Geometry check sheet. Reference: the model listing, model coordinates, mm. Face numbers are marked on the shaded views. Round coordinates to 2 decimals unless told otherwise and drop trailing zeros. Loops run counter-clockwise (first coordinate to the right, second up) from the corner with the lowest first, then second, coordinate; pieces in that order, holes last. Notation, with made-up numbers: M -40,77 L 8,77 A27 cw 8,96 Z; hole C 6.25,62 d5. An arc over 180 degrees is marked long. Write item = value, one per line.
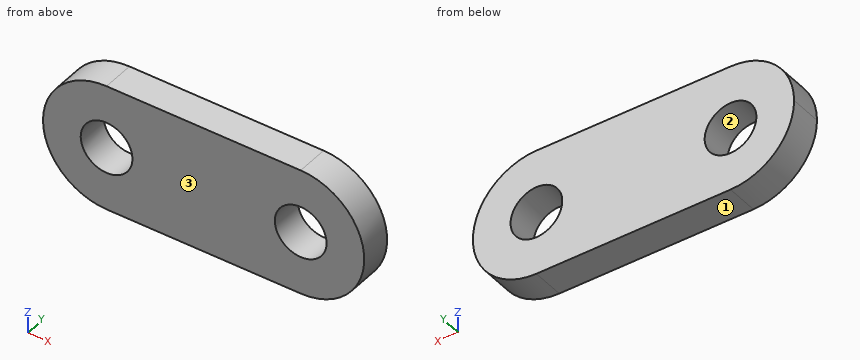
from build123d import *

# Parameters (mm, degrees)
F0_R     = 4.0005
F1_DEPTH = 2.5


with BuildPart() as f1:
    # F0 (on Front) → F1 (new body, symmetric)
    with BuildSketch(Plane.XZ):
        with BuildLine():
            Line((0, 9.8298), (0, 0))
            Line((0, 0), (-11.0109, 0))
            ThreePointArc((-11.0109, 0), (-15.0114, -4.0005), (-19.0119, 0))
            Line((-19.0119, 0), (-24.8412, 0))
            ThreePointArc((-24.8412, 0), (-21.962118, -6.950718), (-15.0114, -9.8298))
            Line((-15.0114, -9.8298), (0, -9.8298))
            Line((0, -9.8298), (15.0114, -9.8298))
            ThreePointArc((15.0114, -9.8298), (24.8412, 0), (15.0114, 9.8298))
            Line((15.0114, 9.8298), (0, 9.8298))
        make_face()
        with Locations((15.0114, 0)):
            Circle(F0_R, mode=Mode.SUBTRACT)
        with BuildLine():
            Line((-11.0109, 0), (0, 0))
            Line((0, 0), (0, 9.8298))
            Line((0, 9.8298), (-15.0114, 9.8298))
            ThreePointArc((-15.0114, 9.8298), (-21.962118, 6.950718), (-24.8412, 0))
            Line((-24.8412, 0), (-19.0119, 0))
            ThreePointArc((-19.0119, 0), (-15.0114, 4.0005), (-11.0109, 0))
        make_face()
    extrude(amount=F1_DEPTH, both=True)


solid = f1.part
(1) Sectioned sample at A-A on y = 0.2. Record the cut outline in (x, z).
Result set:
outline = M -24.84,0 A9.83 ccw -15.01,-9.83 L 15.01,-9.83 A9.83 ccw 15.01,9.83 L -15.01,9.83 A9.83 ccw Z; hole C -15.01,0 d8; hole C 15.01,0 d8
(2) Release check for a two-part mould opening along Z. For the marked faces 1, 2 and 3 record: released by +Z, released by -Z, zero draft, split by the parting line, or undercut.
Result set:
face_1 = released by -Z
face_2 = undercut
face_3 = zero draft
(3) Depth check by flat-ended pin: pin 1 Ø1.5 at (x, y) = (-16, -0.5) entering from -Z. Enter the tip coordinate at first touch or a pass-through.
Result set:
pin_1 = -9.83
(4) Material ranges on line 1 along Z through (x, y) = (-15, -0.4); line 2 along X through (y, z) = (-1.2, 3.5); line 3 along X through (y, z) = (-0.9, 2.5), recorded low to high. Write a range as from..to.
Result set:
line_1 = -9.83..-4, 4..9.83
line_2 = -24.2..-16.95, -13.07..13.07, 16.95..24.2
line_3 = -24.52..-18.13, -11.89..11.89, 18.13..24.52
(5) Sectioned sample at C-C on z = -7.25. Record the cut outline in (x, y), then the cut area to 3 significant figures.
Result set:
outline = M -21.65,-2.5 L 21.65,-2.5 L 21.65,2.5 L -21.65,2.5 Z
area = 216 mm2
(6) Sectioned sample at B-B on x = 20. Record the cut outline in (y, z), then the cut area to 3 significant figures.
Result set:
outline = M -2.5,-8.47 L 2.5,-8.47 L 2.5,8.47 L -2.5,8.47 Z
area = 84.7 mm2
